Check sheet for the modelled part. Datum: model origin and axes. Units: mm. A direction names the side the tool comes from. Give positions to 0.01 mm unless a question says otherwise; leave off trailing zeros. Write each loop counter-clockwise with the first axis right and the second up, starting at its lowest first coordinate (ties: lowest second). Pieces come first, ordered by that corner, then holes. Notation, with made-up numbers: (89.5, -3.75) -> (138.5, -3.75) arc R31 ccw to (138.5, 25.25) -> close; hole circle Ø3 at (-3, 61). An arc over 180 degrees is marked (long way). Return JSON: item names as keys, results as strings.
from build123d import *

# Parameters (mm, degrees)
SKETCH1_W          = 470
SKETCH1_H          = 50
CUT_EXTRUDE1_DEPTH = 20


with BuildPart() as part:
    # Sketch1 → Revolve1 (revolve)
    with BuildSketch(Plane(origin=(0, 0, 0), x_dir=(0, 0, -1), z_dir=(1, 0, 0))):
        with Locations((-265, 0)):
            Rectangle(SKETCH1_W, SKETCH1_H)
    revolve(axis=Axis((0, 285.555555556, 0), (0, -1, 0)))

    # Sketch2 → Cut-Extrude1 (cut)
    with BuildSketch(Plane.XZ.offset(25)):
        with BuildLine():
            Line((-180, 446.476151588), (-122.573000413, 307.835110337))
            ThreePointArc((-122.573000413, 307.835110337), (0, 330), (122.573000413, 307.835110337))
            Line((122.573000413, 307.835110337), (180, 446.476151588))
            ThreePointArc((180, 446.476151588), (0, 480), (-180, 446.476151588))
        make_face()
        with BuildLine():
            Line((188.427093812, 442.985535039), (131.000094225, 304.344493789))
            ThreePointArc((131.000094225, 304.344493789), (233.345237792, 233.345237792), (304.344493789, 131.000094225))
            Line((304.344493789, 131.000094225), (442.985535039, 188.427093812))
            ThreePointArc((442.985535039, 188.427093812), (339.41125497, 339.41125497), (188.427093812, 442.985535039))
        make_face()
        with BuildLine():
            Line((446.476151588, 180), (307.835110337, 122.573000413))
            ThreePointArc((307.835110337, 122.573000413), (330, 0), (307.835110337, -122.573000413))
            Line((307.835110337, -122.573000413), (446.476151588, -180))
            ThreePointArc((446.476151588, -180), (480, 0), (446.476151588, 180))
        make_face()
        with BuildLine():
            Line((442.985535039, -188.427093812), (304.344493789, -131.000094225))
            ThreePointArc((304.344493789, -131.000094225), (233.345237792, -233.345237792), (131.000094225, -304.344493789))
            Line((131.000094225, -304.344493789), (188.427093812, -442.985535039))
            ThreePointArc((188.427093812, -442.985535039), (339.41125497, -339.41125497), (442.985535039, -188.427093812))
        make_face()
        with BuildLine():
            Line((180, -446.476151588), (122.573000413, -307.835110337))
            ThreePointArc((122.573000413, -307.835110337), (0, -330), (-122.573000413, -307.835110337))
            Line((-122.573000413, -307.835110337), (-180, -446.476151588))
            ThreePointArc((-180, -446.476151588), (0, -480), (180, -446.476151588))
        make_face()
        with BuildLine():
            Line((-188.427093812, -442.985535039), (-131.000094225, -304.344493789))
            ThreePointArc((-131.000094225, -304.344493789), (-233.345237792, -233.345237792), (-304.344493789, -131.000094225))
            Line((-304.344493789, -131.000094225), (-442.985535039, -188.427093812))
            ThreePointArc((-442.985535039, -188.427093812), (-339.41125497, -339.41125497), (-188.427093812, -442.985535039))
        make_face()
        with BuildLine():
            Line((-446.476151588, -180), (-307.835110337, -122.573000413))
            ThreePointArc((-307.835110337, -122.573000413), (-330, 0), (-307.835110337, 122.573000413))
            Line((-307.835110337, 122.573000413), (-446.476151588, 180))
            ThreePointArc((-446.476151588, 180), (-480, 0), (-446.476151588, -180))
        make_face()
        with BuildLine():
            Line((-442.985535039, 188.427093812), (-304.344493789, 131.000094225))
            ThreePointArc((-304.344493789, 131.000094225), (-233.345237792, 233.345237792), (-131.000094225, 304.344493789))
            Line((-131.000094225, 304.344493789), (-188.427093812, 442.985535039))
            ThreePointArc((-188.427093812, 442.985535039), (-339.41125497, 339.41125497), (-442.985535039, 188.427093812))
        make_face()
    extrude(amount=-CUT_EXTRUDE1_DEPTH, mode=Mode.SUBTRACT)


solid = part.part
(1) Set-up check for faces 1 (the cylindrical face through (-479.993, -15.14, 2.578)), 2 (the flat face through (104, -25, -7)): record each of +Z, -Z, +X, -X, +Y, -Y from which the full face is reachable in a straight line by a thin tool's end or side.
Reply:
{"face 1": "-Y", "face 2": "+Z, -Z, +X, -X, -Y"}
(2) Release check for a two-part mould opening along Z. For faces 3 (the flat face through (-3, -5, -393)), 4 (the flat face through (104, 25, -7)) record: pulls with the +Z half, pulls with the -Z half, needs draft (parallel to the pull), parting line crosses it, or undercut.
Reply:
{"face 3": "undercut", "face 4": "needs draft"}
(3) Cross-section at D-D on x = -359.5. Enter the section's corners in (y, z).
Reply:
{"outline": "(-25, -347.51) -> (25, -347.51) -> (25, 347.51) -> (-25, 347.51) -> (-25, 318.11) -> (-5, 318.11) -> (-5, 153.85) -> (-25, 153.85) -> (-25, 143.97) -> (-5, 143.97) -> (-5, -143.97) -> (-25, -143.97) -> (-25, -153.85) -> (-5, -153.85) -> (-5, -318.11) -> (-25, -318.11) -> close"}
(4) Thickness scan on L1, parallel to Z at x = 0, y = 14; L2, parallel to Z at x = -39, y = -11.5; L3, parallel to Z at x = 273, y = -16.5. Record the ranges inside material, lowest first.
Reply:
{"L1": "-500 to -30, 30 to 500", "L2": "-498.48 to -478.48, -327.82 to 327.82, 478.48 to 498.48", "L3": "-418.89 to -395.19, -185.98 to 185.98, 395.19 to 418.89"}
(5) Depth check by flat-ended pin: pin 1 Ø5 at (x, y) = (304, 6) entering from -Z; pin 2 Ø4 at (x, z) = (-378.5, 167) entering from -Y; pin 3 Ø1 at (x, y) = (297.5, 0) entering from -Z. Enter the tip coordinate at first touch or a pass-through.
Reply:
{"pin 1": "z = -398.87", "pin 2": "y = -5", "pin 3": "z = -402.23"}
(6) Cross-section at A-A on x = 0. Enter the section's corners in (y, z).
Reply:
{"outline": "(-25, -500) -> (25, -500) -> (25, -30) -> (-25, -30) -> (-25, -330) -> (-5, -330) -> (-5, -480) -> (-25, -480) -> close; (-25, 30) -> (25, 30) -> (25, 500) -> (-25, 500) -> (-25, 480) -> (-5, 480) -> (-5, 330) -> (-25, 330) -> close"}
(7) Cross-section at B-B on z = 0. Enter the section's corners in (x, y), then the cut area to 3 significant figures.
Reply:
{"outline": "(-500, -25) -> (-480, -25) -> (-480, -5) -> (-330, -5) -> (-330, -25) -> (-30, -25) -> (-30, 25) -> (-500, 25) -> close; (30, -25) -> (330, -25) -> (330, -5) -> (480, -5) -> (480, -25) -> (500, -25) -> (500, 25) -> (30, 25) -> close", "area": "41,000 mm^2"}
(8) Cross-section at C-C on y = 7. Enter the section's corners in (x, z), then the cut area to 3 significant figures.
Reply:
{"outline": "circle Ø1000 at (0, 0); hole circle Ø60 at (0, 0)", "area": "783,000 mm^2"}
